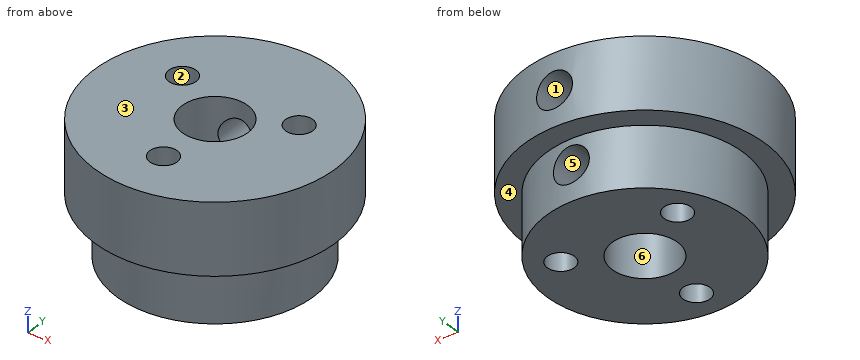
```python
from build123d import *

# Parameters (mm, degrees)
M3X0_5_TAPPED_HOLE1_D               = 2.5
M4X0_7_TAPPED_HOLE1_D               = 3.3
M4X0_7_TAPPED_HOLE1_DEPTH           = 10.999
M4X0_7_TAPPED_HOLE1_TIP             = 0.991420021
M4X0_7_TAPPED_HOLE1_ON_FACE_2_D     = 3.3
M4X0_7_TAPPED_HOLE1_ON_FACE_2_DEPTH = 10.999
M4X0_7_TAPPED_HOLE1_ON_FACE_2_TIP   = 0.991420021


with BuildPart() as part:
    # Sketch2 → Revolve1 (revolve)
    with BuildSketch(Plane(origin=(0, 0, 0), x_dir=(0, 0, -1), z_dir=(1, 0, 0)), mode=Mode.PRIVATE) as revolve1_sk:
        Polygon((0, 3), (0, 11), (6.5, 11), (6.5, 9), (12, 9), (12, 3), align=None)
    revolve(revolve1_sk.sketch.rotate(Axis((0, 0, 0), (0, 0, -1)), 90), axis=Axis((0, 0, 0), (0, 0, -1)))

    # M3x0.5 Tapped Hole1 (through all)
    with Locations(Plane.XY):
        with Locations((35.910466859, 13.470944302), (5.369357503, 3.1), (-5.369357503, 3.1), (0, -6.2)):
            Hole(M3X0_5_TAPPED_HOLE1_D / 2)

    # M4x0.7 Tapped Hole1
    with Locations(Plane(origin=(0, 9, -8.75), x_dir=(1, 0, 0), z_dir=(0, 1, 0))):
        with Locations((0, 0)):
            Hole(M4X0_7_TAPPED_HOLE1_D / 2, depth=M4X0_7_TAPPED_HOLE1_DEPTH)
            with Locations((0, 0, -(M4X0_7_TAPPED_HOLE1_DEPTH + M4X0_7_TAPPED_HOLE1_TIP / 2))):  # 118° drill point
                Cone(0, M4X0_7_TAPPED_HOLE1_D / 2, M4X0_7_TAPPED_HOLE1_TIP, mode=Mode.SUBTRACT)

    # M4x0.7 Tapped Hole1 on face 2
    with Locations(Plane(origin=(0, 11, -3.25), x_dir=(0, 0, 1), z_dir=(0, 1, 0))):
        with Locations((0, 0)):
            Hole(M4X0_7_TAPPED_HOLE1_ON_FACE_2_D / 2, depth=M4X0_7_TAPPED_HOLE1_ON_FACE_2_DEPTH)
            with Locations((0, 0, -(M4X0_7_TAPPED_HOLE1_ON_FACE_2_DEPTH + M4X0_7_TAPPED_HOLE1_ON_FACE_2_TIP / 2))):  # 118° drill point
                Cone(0, M4X0_7_TAPPED_HOLE1_ON_FACE_2_D / 2, M4X0_7_TAPPED_HOLE1_ON_FACE_2_TIP, mode=Mode.SUBTRACT)


solid = part.part
```
Geometry: final body of the model. Coordinates: model frame, mm. Face numbers are marked on the shaded views. A direction names the side the tool comes from. Round coordinates to 2 decimals unless told otherwise and drop trailing zeros. Write each loop counter-clockwise with the first axis right and the second up, starting at its lowest first coordinate (ties: lowest second). Pieces come first, ordered by that corner, then holes. Notation, with made-up numbers: M 43.5,88 L 78.5,88 A16 cw 78.5,116 Z; hole C 69.25,14 d8. An arc over 180 degrees is marked long. Answer in a Markdown table with one row per item. Add a question column.
(1) Cut plane C-C, the plane z = -1.25. Return the cut outline in (x, y), then the cut area to 3 significant figures.
(2) Cut plane D-D, the plane y = 7.75. Return the cut outline in (x, z), then the cut area to 3 significant figures.
(3) Cut plane B-B, the plane y = 0. Return the cut outline in (x, z), then the cut area to 3 significant figures.
(4) Reachability of the marked faces 4, 5 and 6 from +Z, -Z, +X, -X, +Y, -Y: full face, straight path, thin tool, end or side. Return the list, or none.
(5) Draft query along Z for the marked faces 1, 2 and 3. Return one class per face: pulls with the +Z half, pulls with the -Z half, needs draft (parallel to the pull), parting line crosses it, or undercut.
(6) Contact query for flat-ended pins moving along their axis: pin 1 (6 mm diameter, centred on y = 6.5, z = -2, fed in from +X); pin 2 (1.5 mm diameter, centred on y = 8, z = -5.5, fed in from -X); pin 3 (6 mm diameter, centred on y = -3.5, z = -7.5, fed in from -X). Output: stop coordinate, or through.
(7) Cut plane A-A, the plane x = 0. Return the cut outline in (y, z), then the cut area to 3 significant figures.
(8) Ray query, L1, parallel to Z at x = 0, y = 6.75; L2, parallel to X at y = 4, z = -7; L3, parallel to X at y = 2, z = -4.75. Return the intervals inside material, ascending.
Established:
| question | item | result |
|---|---|---|
| 1 | outline | C 0,0 d22; hole C -5.37,3.1 d2.5; hole C 0,0 d6; hole C 0,-6.2 d2.5; hole C 5.37,3.1 d2.5 |
| 1 | area | 337 mm² |
| 2 | outline | M -7.81,-6.5 L -4.58,-6.5 L -4.58,-12 L 4.58,-12 L 4.58,-6.5 L 7.81,-6.5 L 7.81,0 L -7.81,0 Z; hole C 0,-8.75 d3.3; hole C 0,-3.25 d3.3 |
| 2 | area | 135 mm² |
| 3 | outline | M -11,-6.5 L -9,-6.5 L -9,-12 L -3,-12 L -3,0 L -11,0 Z; M 3,-12 L 9,-12 L 9,-6.5 L 11,-6.5 L 11,0 L 3,0 Z |
| 3 | area | 170 mm² |
| 4 | face 4 | -Z |
| 4 | face 5 | +Y |
| 4 | face 6 | +Z, -Z |
| 5 | face 1 | undercut |
| 5 | face 2 | needs draft |
| 5 | face 3 | pulls with the +Z half |
| 6 | pin 1 | x = 10.43 |
| 6 | pin 2 | x = -8.27 |
| 6 | pin 3 | x = -10.98 |
| 7 | outline | M -11,-6.5 L -9,-6.5 L -9,-12 L -7.45,-12 L -7.45,0 L -11,0 Z; M -4.95,-12 L -3,-12 L -3,0 L -4.95,0 Z; M 3,-12 L 9,-12 L 9,-10.4 L 3,-10.4 Z; M 3,-7.1 L 9,-7.1 L 9,-6.5 L 11,-6.5 L 11,-4.9 L 3,-4.9 Z; M 3,-1.6 L 11,-1.6 L 11,0 L 3,0 Z |
| 7 | area | 93.8 mm² |
| 8 | L1 | -12 to -10.4, -7.1 to -4.9, -1.6 to 0 |
| 8 | L2 | -8.06 to -6.24, -4.5 to 4.5, 6.24 to 8.06 |
| 8 | L3 | -10.82 to -5.96, -4.78 to -2.24, 2.24 to 4.78, 5.96 to 10.82 |
